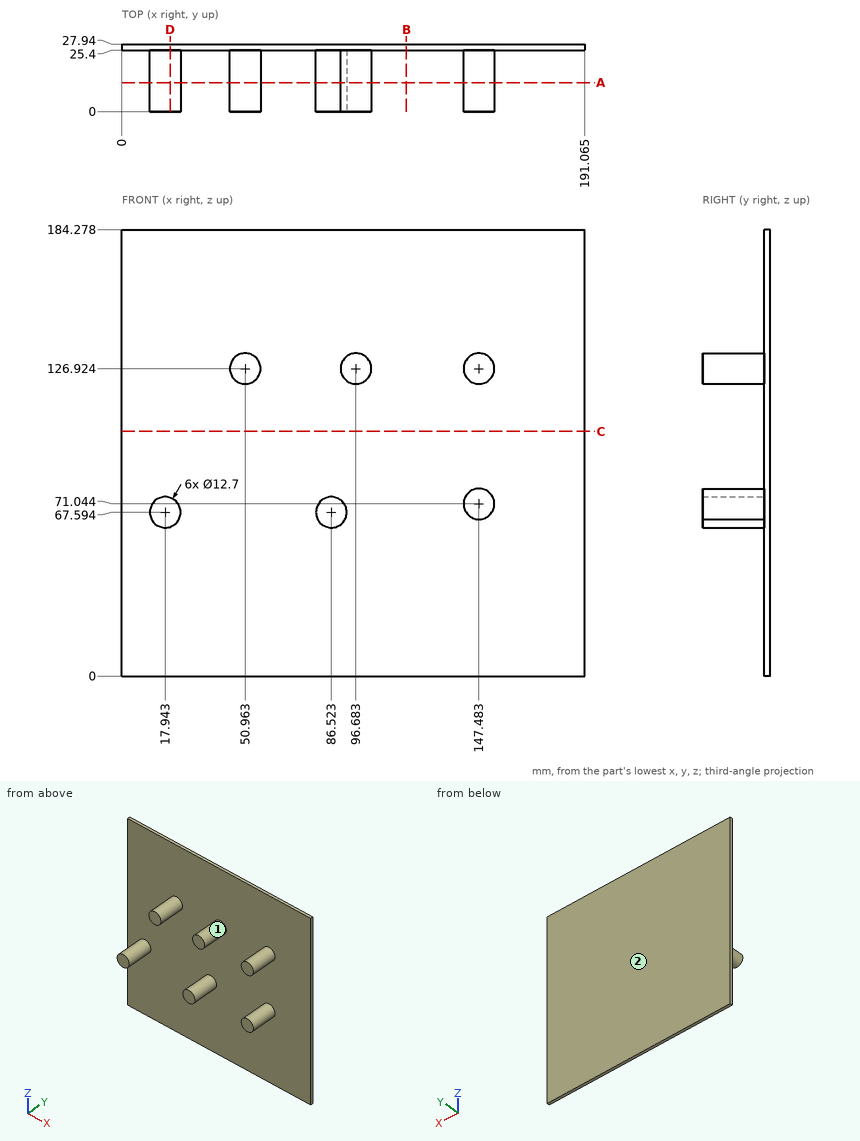
Answer from the drawing. Dimensions are ordinates in mm from the lowest x, y and z of the part. Give positions to 0.01 mm unless a question says otherwise; leave off trailing zeros. Write each loop counter-clockwise with the first axis right and the second up, starting at its lowest first coordinate (ties: lowest second). Pieces come first, ordered by that corner, then holes. Notation, with made-up numbers: (9.25, -22.5) - (18.25, -22.5) arc R9 cw to (18.25, -18.5) - close; hole circle Ø3 at (56, 44). An arc over 180 degrees is marked (long way). Answer in a Markdown table with one row per item. Add a question column.
Item 1: Flat-ended cylindrical pins translate along their axes: P1, Ø5, axis at x = 100.5, y = 3, coming from the +Z side; P2, Ø4, axis at x = 129.5, z = 108, coming from the -Y side. Find the tip coordinate at first contact, or state that the pin passes through.
Item 2: Section B-B, the plane x = 117.5 is taken. Write down the section's boundary in (y, z).
Item 3: Section C-C, the plane z = 101 is taken. Write down the section's boundary in (x, y) (1 decimal).
Item 4: Section A-A, the plane y = 12 is taken. Count the separate pieces of the cut face and the enclosed holes in it, and give its area (3 significant figures).
Item 5: Section D-D, the plane x = 20 is taken. Write down the section's boundary in (y, z).
Item 6: Determine the mould class of the marked faces 1 and 2 for opening direction X: pulls with the +X half, pulls with the -X half, needs draft (parallel to the pull), parting line crosses it, or undercut.
Item 7: Find the intervals of material crossed by L1, parallel to Y at x = 94.5, z = 141; L2, parallel to X at y = 21.75, z = 73 (1 decimal); L3, parallel to Z at x = 144.5, y = 2, in increasing order.
Recorded:
| question | item | result |
|---|---|---|
| 1 | P1 | stops at z = 133.14 |
| 1 | P2 | stops at y = 25.4 |
| 2 | outline | (25.4, 0) - (27.94, 0) - (27.94, 184.28) - (25.4, 184.28) - close |
| 3 | outline | (0, 25.4) - (191.1, 25.4) - (191.1, 27.9) - (0, 27.9) - close |
| 4 | separate pieces | 6 |
| 4 | enclosed holes | 0 |
| 4 | area | 760 mm2 |
| 5 | outline | (0, 61.59) - (25.4, 61.59) - (25.4, 0) - (27.94, 0) - (27.94, 184.28) - (25.4, 184.28) - (25.4, 73.6) - (0, 73.6) - close |
| 6 | face 1 | undercut |
| 6 | face 2 | needs draft |
| 7 | L1 | y = 25.4 to 27.94 |
| 7 | L2 | x = 14.6 to 21.3, 83.2 to 89.9, 141.4 to 153.5 |
| 7 | L3 | z = 65.44 to 76.65, 121.32 to 132.53 |
